The model under review builds one solid part; all positions refer to its coordinate system, in mm. Give positions to 0.01 mm unless a question says otherwise; leave off trailing zeros. Loops run counter-clockwise (first coordinate to the right, second up) from the corner with the lowest first, then second, coordinate; pieces in that order, holes last. Notation, with made-up numbers: (41.5, 22) - (52.5, 22) arc R14 ccw to (52.5, 27) - close; hole circle Ø7 at (0.25, 25.5). An arc over 180 degrees is marked (long way). Return JSON: item names as keys, results as strings. Group by question number.
Solid Edge part; units mm, degrees
sketch "Sketch1" plane through (0, 0, 0) normal (0, -1, 0) x (1, 0, 0)
  circle A0 centre (0, 0) radius 40.5
extrude "Protrusion1" add sketch "Sketch1" along normal mid plane 100
sketch "Sketch2" plane through (0, 0, 0) normal (0, -1, 0) x (1, 0, 0)
  circle A0 centre (0, 0) radius 39
extrude "ExtrudedCutout_1" cut sketch "Sketch2" along normal mid plane 100
sketch "Sketch3" plane through (0, 0, 0) normal (1, 0, 0) x (0, 1, 0)
  circle A0 centre (-25, 0) radius 4
extrude "Cutout1" cut sketch "Sketch3" along normal mid plane 85
sketch "Sketch4" plane through (0, 0, 0) normal (1, 0, 0) x (0, 1, 0)
  circle A0 centre (25, 0) radius 4
extrude "ExtrudedCutout_5" cut sketch "Sketch4" along normal mid plane 85
1) To check wall thickness, follow line 1 (Y direction, x = 39.8, z = 0); line 2 (X direction, y = 7, z = 0); line 3 (Z direction, x = -1, y = -20). State the ranges of each line that lie inside material, in increasing order.
2) We need section C-C, the plane z = 0. Write out the cut boundary in (x, y), plus the area to 3 significant figures.
3) We need section A-A, the plane x = 0. Write out the cut boundary in (y, z).
4) We need section B-B, the plane y = -25. Write out the cut boundary in (x, z).
5) We need section D-D, the plane y = 12. Write out the cut boundary in (x, z), plus the area to 3 significant figures.
6) Draft analysis for pull direction Z (two halves, no side actions). For faces 1 (the face through (38.63, 0.7, -12.17)), 2 (the face through (40, 21, 0)), 3 (the face through (33.2, 50, 21.2)), state which applies: +Z half, -Z half, draft (parallel to the pull), parting line (faces both ways), or undercut.
7) For pin 1 Ø10.5 at (y, z) = (-25, 0) entering from +X; pin 2 Ø3 at (x, y) = (12.5, -16) entering from -Z; pin 3 Ø10 at (x, y) = (-5, 38) entering from -Z; pin 4 Ø1.5 at (x, y) = (31.5, 27) entering from +Z, all flat-tipped, find the tip position at first contact; note any pin that passes through.
Findings:
{
 "1": {"line 1": "y = -50 to -29, -21 to 21, 29 to 50", "line 2": "x = -40.5 to -39, 39 to 40.5", "line 3": "z = -40.49 to -38.99, 38.99 to 40.49"},
 "2": {"outline": "(-40.5, -50) - (-39, -50) - (-39, -29) - (-40.5, -29) - close; (-40.5, -21) - (-39, -21) - (-39, 21) - (-40.5, 21) - close; (-40.5, 29) - (-39, 29) - (-39, 50) - (-40.5, 50) - close; (39, -50) - (40.5, -50) - (40.5, -29) - (39, -29) - close; (39, -21) - (40.5, -21) - (40.5, 21) - (39, 21) - close; (39, 29) - (40.5, 29) - (40.5, 50) - (39, 50) - close", "area": "252 mm^2"},
 "3": {"outline": "(-50, -40.5) - (50, -40.5) - (50, -39) - (-50, -39) - close; (-50, 39) - (50, 39) - (50, 40.5) - (-50, 40.5) - close"},
 "4": {"outline": "(-40.3, -4) arc R40.5 ccw to (40.3, -4) - (38.79, -4) arc R39 cw to (-38.79, -4) - close; (-40.3, 4) - (-38.79, 4) arc R39 cw to (38.79, 4) - (40.3, 4) arc R40.5 ccw to start"},
 "5": {"outline": "circle Ø81 at (0, 0); hole circle Ø78 at (0, 0)", "area": "375 mm^2"},
 "6": {"face 1": "parting line", "face 2": "undercut", "face 3": "draft"},
 "7": {"pin 1": "stops at x = 40.5", "pin 2": "stops at z = -38.98", "pin 3": "stops at z = -40.5", "pin 4": "stops at z = 26.36"}
}
